Print and shaded views of the part. All mm, measured from the part's lowest x, y and z. A direction names the side the tool comes from. Round coordinates to 2 decimals unless told otherwise and drop trailing zeros. Loops run counter-clockwise (first coordinate to the right, second up) from the corner with the lowest first, then second, coordinate; pieces in that order, holes last. Notation, with made-up numbers: (0.5, 35) - (33.5, 35) arc R28 cw to (33.5, 61) - close; hole circle Ø3 at (2.25, 58.5). An arc over 180 degrees is marked (long way). Answer as a JSON object with one key per item and string values.
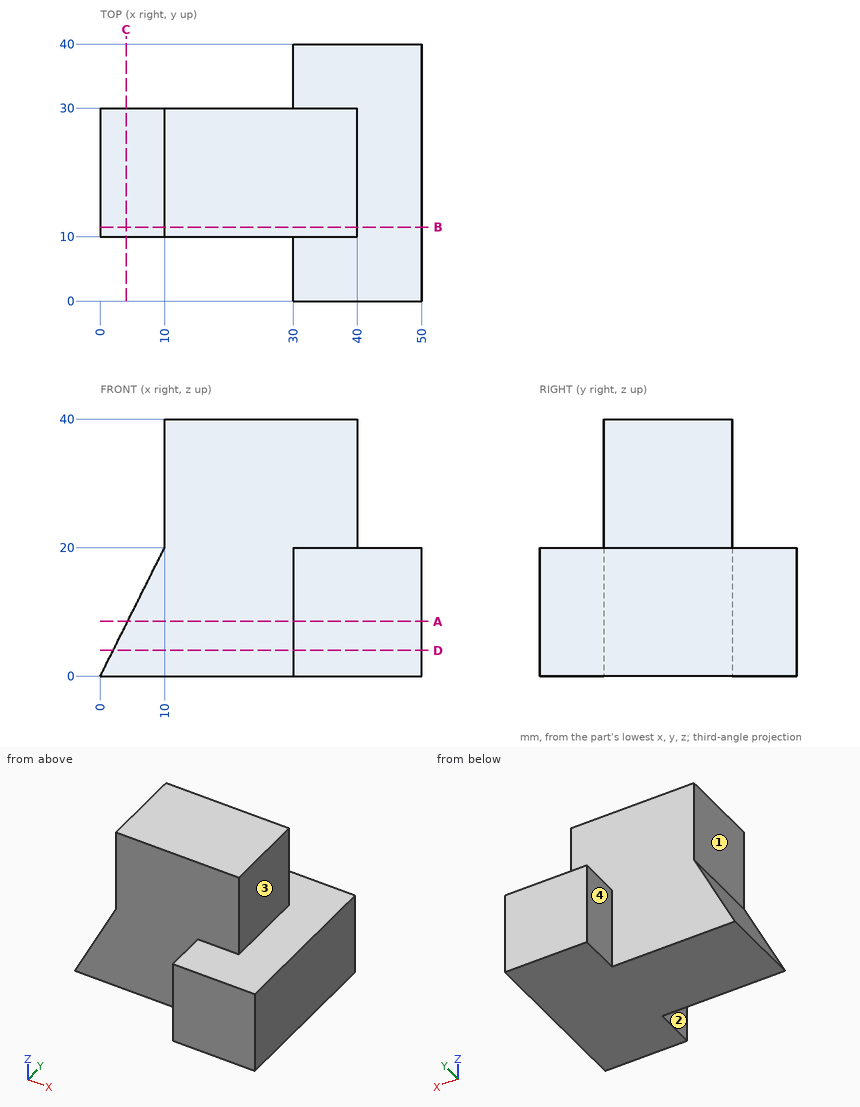
1) Slice it at C-C on x = 4. List the corners of the cut face in (y, z), then the cut area to 3 significant figures.
Values follow:
{"outline": "(10, 0) - (30, 0) - (30, 8) - (10, 8) - close", "area": "160 mm²"}
2) Slice it at D-D on z = 4. List the corners of the cut face in (x, y), then the cut area to 3 significant figures.
Values follow:
{"outline": "(2, 10) - (30, 10) - (30, 0) - (50, 0) - (50, 40) - (30, 40) - (30, 30) - (2, 30) - close", "area": "1,360 mm²"}
3) Probe probe 1 along Z at (x, y) = (44.5, 18); probe 2 along X at (y, z) = (17, 23); probe 3 along Y at (x, z) = (22.5, 9). List the from-to ranges inside material, lowest first.
Values follow:
{"probe 1": "0 to 20", "probe 2": "10 to 40", "probe 3": "10 to 30"}
4) Slice it at B-B on y = 11.5. List the corners of the cut face in (x, z), then the cut area to 3 significant figures.
Values follow:
{"outline": "(0, 0) - (50, 0) - (50, 20) - (40, 20) - (40, 40) - (10, 40) - (10, 20) - close", "area": "1,500 mm²"}
5) Slice it at A-A on z = 8.5. List the corners of the cut face in (x, y), then the cut area to 4 significant figures.
Values follow:
{"outline": "(4.25, 10) - (30, 10) - (30, 0) - (50, 0) - (50, 40) - (30, 40) - (30, 30) - (4.25, 30) - close", "area": "1,315 mm²"}
6) Tool access for the marked faces 1, 2, 3 and 4: list every direction of +Z, -Z, +X, -X, +Y, -Y with a clear straight run to the whole face (end or side of a thin tool).
Values follow:
{"face 1": "+Z, -X, +Y, -Y", "face 2": "+Z, -Z, -X, -Y", "face 3": "+Z, +X, +Y, -Y", "face 4": "+Z, -Z, -X, +Y"}
7) Drop flat-ended pins along their axis: P1, Ø1, axis at y = 18.5, z = 21.5, coming from the -X side; P2, Ø8, axis at x = 8, z = 34, coming from the +Y side; P3, Ø16, axis at y = 21, z = 33, coming from the +X side. Give the stop position or say it passes through.
Values follow:
{"P1": "x = 10", "P2": "y = 30", "P3": "x = 40"}
